Could you check a few things on this model? Use its own coordinates, in mm. Face numbers are marked on the shaded views. Round coordinates to 2 decimals unless told otherwise and drop trailing zeros. Write each loop counter-clockwise with the first axis right and the second up, starting at its lowest first coordinate (ties: lowest second). Pieces come first, ordered by that corner, then holes. Notation, with made-up numbers: (29, -33) -> (52, -33) arc R15 cw to (52, -22) -> close; hole circle Ø11 at (-29, 28). An arc over 180 degrees is marked (long way). One line per question, with ' | ' between items. Start each with the question number.
1. Imagine slicing it at A-A, the plane x = -230.5. List the corners of the cut face in (y, z) for me, and give its area (3 significant figures).
2. If I drill on line 1 along Y through (x, z) = (-71.5, 598.5); line 2 along X through (y, z) = (21.5, 623); line 3 along Z through (x, y) = (-294, 126), over which ranges is the centre line in solid material (lowest first)? Write a range as [from, to].
3. For pin 1 Ø16 at (y, z) = (22.5, 621) entering from +X; pin 2 Ø1 at (x, y) = (-284, 124) entering from +Z; pin 3 Ø10 at (y, z) = (24, 626) entering from -X; pin 4 Ø25 at (x, z) = (-245.5, 622) entering from +Y, each with a flat end and sliding along its axis, tell me the tip position at first contact or that it passes through.
4. Imagine slicing it at C-C, the plane x = -67. List the corners of the cut face in (y, z) for me, and give its area (3 significant figures).
5. Thinking about a two-plate mould opening in Y: for the marked faces 1, 2 and 3, which applies, released by +Y, released by -Y, zero draft, split by the parting line, or undercut?
6. Imagine slicing it at B-B, the plane y = 234. List the corners of the cut face in (x, z) for me.
7. Imagine slicing it at D-D, the plane x = -370. List the corners of the cut face in (y, z) for me, and give its area (3 significant figures).
from build123d import *

# Parameters (mm, degrees)
SKETCH_1_W          = 400
SKETCH_1_H          = 600
EXTRUDE_1_DEPTH     = 300
SKETCH_2_W          = 200
SKETCH_2_H          = 20
EXTRUDE_2_DEPTH     = 50
SKETCH_3_W          = 180
SKETCH_3_H          = 35
CUT_EXTRUDE_1_DEPTH = 50
SKETCH_4_W          = 320
SKETCH_4_H          = 220
CUT_EXTRUDE_2_DEPTH = 2


with BuildPart() as part:
    # Эскиз1 → Бобышка-Вытянуть1 (new body)
    with BuildSketch(Plane(origin=(0, 0, 0), x_dir=(1, 0, 0), z_dir=(0, 1, 0))):
        with Locations((-200, -300)):
            Rectangle(SKETCH_1_W, SKETCH_1_H)
    extrude(amount=EXTRUDE_1_DEPTH)

    # Эскиз2 → Бобышка-Вытянуть2 (add)
    with BuildSketch(Plane.XY.offset(600)):
        with Locations((-200, 25)):
            Rectangle(SKETCH_2_W, SKETCH_2_H)
    extrude(amount=EXTRUDE_2_DEPTH)

    # Эскиз3 → Вырез-Вытянуть1 (cut)
    with BuildSketch(Plane(origin=(0, 35, 0), x_dir=(1, 0, 0), z_dir=(0, 1, 0))):
        with Locations((-200, -625)):
            Rectangle(SKETCH_3_W, SKETCH_3_H)
    extrude(amount=-CUT_EXTRUDE_1_DEPTH, mode=Mode.SUBTRACT)

    # Эскиз4 → Вырез-Вытянуть2 (cut)
    with BuildSketch(Plane.XY.offset(600)):
        with Locations((-200, 150)):
            Rectangle(SKETCH_4_W, SKETCH_4_H)
    extrude(amount=-CUT_EXTRUDE_2_DEPTH, mode=Mode.SUBTRACT)


solid = part.part
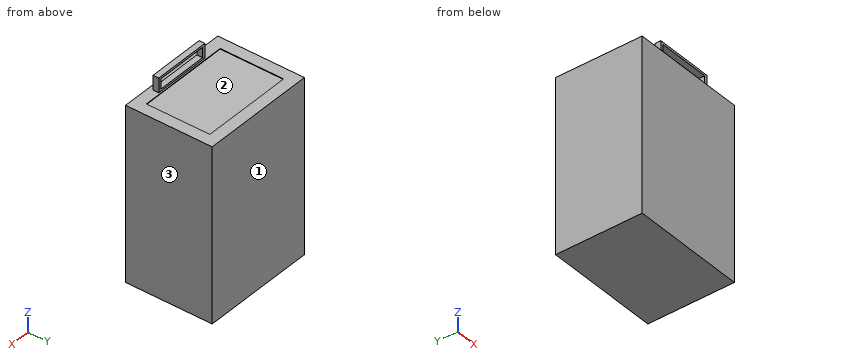
Geometry results:
1) outline: (0, 0) -> (300, 0) -> (300, 600) -> (260, 600) -> (260, 598) -> (40, 598) -> (40, 600) -> (35, 600) -> (35, 607.5) -> (15, 607.5) -> (15, 600) -> (0, 600) -> close; (15, 642.5) -> (35, 642.5) -> (35, 650) -> (15, 650) -> close | area: 180,000 mm2
2) line 1: y = [0, 40], [260, 300] | line 2: x = [-300, -290], [-110, -100] | line 3: z = [0, 598]
3) pin 1: stops at x = -100 | pin 2: stops at z = 598 | pin 3: stops at x = -300 | pin 4: passes through
4) outline: (0, 0) -> (300, 0) -> (300, 600) -> (260, 600) -> (260, 598) -> (40, 598) -> (40, 600) -> (0, 600) -> close | area: 180,000 mm2
5) face 1: released by +Y | face 2: undercut | face 3: zero draft
6) outline: (-400, 0) -> (0, 0) -> (0, 600) -> (-40, 600) -> (-40, 598) -> (-360, 598) -> (-360, 600) -> (-400, 600) -> close
7) outline: (0, 0) -> (300, 0) -> (300, 600) -> (0, 600) -> close | area: 180,000 mm2
